The listing builds one solid part. Answer for the finished solid, in the listing's coordinates (mm). Face numbers are marked on the shaded views. A direction names the side the tool comes from. Coordinates: 2 decimals unless noted, no trailing zeros. Write each loop counter-clockwise with the first axis right and the second up, starting at its lowest first coordinate (ties: lowest second). Pieces come first, ordered by that corner, then holes. Notation, with made-up numbers: M 79.5,27.25 L 103.5,27.25 A19 cw 103.5,35.25 Z; hole C 67.25,-9.5 d10. An arc over 180 degrees is marked long. Answer as a JSON object with one key per item and string values. Group by question number.
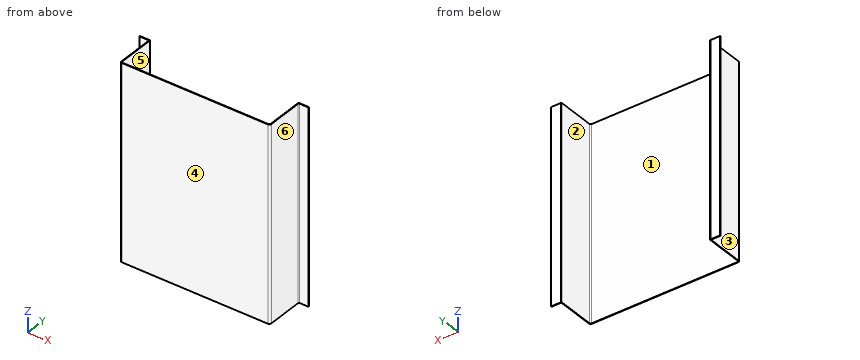
from build123d import *

# Parameters (mm, degrees)
BOSS_EXTRUDE1_DEPTH = 475.488


with BuildPart() as part:
    # Sketch2 → Boss-Extrude1 (new body)
    with BuildSketch(Plane.XY):
        with BuildLine():
            Line((-179.1462, 0), (179.1462, 0))
            ThreePointArc((179.1462, 0), (182.504815789, 1.391184211), (183.896, 4.7498))
            Line((183.896, 4.7498), (183.896, 93.6625))
            ThreePointArc((183.896, 93.6625), (184.360967985, 94.785032015), (185.4835, 95.25))
            Line((185.4835, 95.25), (207.6958, 95.25))
            Line((207.6958, 95.25), (207.6958, 96.8502))
            Line((207.6958, 96.8502), (183.8833, 96.8502))
            ThreePointArc((183.8833, 96.8502), (182.760767985, 96.385232015), (182.2958, 95.2627))
            Line((182.2958, 95.2627), (182.2958, 4.7625))
            ThreePointArc((182.2958, 4.7625), (181.36586403, 2.51743597), (179.1208, 1.5875))
            Line((179.1208, 1.5875), (-179.1208, 1.5875))
            ThreePointArc((-179.1208, 1.5875), (-181.36586403, 2.51743597), (-182.2958, 4.7625))
            Line((-182.2958, 4.7625), (-182.2958, 95.25))
            Line((-182.2958, 95.25), (-182.2958, 95.2627))
            ThreePointArc((-182.2958, 95.2627), (-182.760767985, 96.385232015), (-183.8833, 96.8502))
            Line((-183.8833, 96.8502), (-207.6958, 96.8502))
            Line((-207.6958, 96.8502), (-207.6958, 95.25))
            Line((-207.6958, 95.25), (-185.4835, 95.25))
            ThreePointArc((-185.4835, 95.25), (-184.360967985, 94.785032015), (-183.896, 93.6625))
            Line((-183.896, 93.6625), (-183.896, 4.7498))
            ThreePointArc((-183.896, 4.7498), (-182.504815789, 1.391184211), (-179.1462, 0))
        make_face()
    extrude(amount=BOSS_EXTRUDE1_DEPTH)


solid = part.part
Item 1: A tool of negligible diameter and unlimited length cuts with its end or side. For the marked faces 5 and 6, from which of +Z, -Z, +X, -X, +Y, -Y can it reach the whole face along a straight path? Write none if from no direction.
Item 2: For a pull along X with two mould halves and no side action, classify the marked faces 1, 2, 3 and 4 as +X half, -X half, draft (parallel to the pull), parting line (faces both ways), or undercut.
Item 3: Flat-ended cylindrical pins translate along their axes: pin 1 Ø1 at (x, z) = (9, 82) entering from +Y; pin 2 Ø11 at (x, z) = (193.5, 312) entering from -Y; pin 3 Ø1 at (y, z) = (64, 353.5) entering from -X. Find the tip coordinate at first contact, or state that the pin passes through.
Item 4: A cutting plane is placed at C-C, the plane x = -140.5. Write down the section's boundary in (y, z), and give its area (3 significant figures).
Item 5: A cutting plane is placed at A-A, the plane y = 82. Write down the section's boundary in (x, z), and give its area (3 significant figures).
Item 6: Consider L1, parallel to X at y = 87.5, z = 290; L2, parallel to Y at x = 38.5, z = 77. Determine where each line is inside the solid, lowest interval first. Write a range as from..to.
Answer:
{
 "1": {"face 5": "+Z, -Z, +Y", "face 6": "+Z, -Z, +X, -Y"},
 "2": {"face 1": "undercut", "face 2": "undercut", "face 3": "-X half", "face 4": "draft"},
 "3": {"pin 1": "y = 1.59", "pin 2": "y = 95.25", "pin 3": "x = -183.9"},
 "4": {"outline": "M 0,0 L 1.59,0 L 1.59,475.49 L 0,475.49 Z", "area": "755 mm2"},
 "5": {"outline": "M -183.9,0 L -182.3,0 L -182.3,475.49 L -183.9,475.49 Z; M 182.3,0 L 183.9,0 L 183.9,475.49 L 182.3,475.49 Z", "area": "1,520 mm2"},
 "6": {"L1": "-183.9..-182.3, 182.3..183.9", "L2": "0..1.59"}
}
